```python
from build123d import *

# Parameters (mm, degrees)
SKETCH1_R           = 1.65
SKETCH1_R_2         = 9.5
BOSS_EXTRUDE1_DEPTH = 1


with BuildPart() as part:
    # Sketch1 → Boss-Extrude1 (new body)
    with BuildSketch(Plane.XY):
        with BuildLine():
            ThreePointArc((10.142857143, 9.649997356), (9, 15.588457268), (3.285714286, 13.608970631))
            ThreePointArc((3.285714286, 13.608970631), (-7, 12.124355653), (-13.428571429, 3.958973274))
            ThreePointArc((-13.428571429, 3.958973274), (-18, 0), (-13.428571429, -3.958973274))
            ThreePointArc((-13.428571429, -3.958973274), (-7, -12.124355653), (3.285714286, -13.608970631))
            ThreePointArc((3.285714286, -13.608970631), (9, -15.588457268), (10.142857143, -9.649997356))
            ThreePointArc((10.142857143, -9.649997356), (14, 0), (10.142857143, 9.649997356))
        make_face()
        with Locations((7, 12.124355653)):
            Circle(SKETCH1_R, mode=Mode.SUBTRACT)
        with Locations((7, -12.124355653)):
            Circle(SKETCH1_R, mode=Mode.SUBTRACT)
        with Locations((-14, 0)):
            Circle(SKETCH1_R, mode=Mode.SUBTRACT)
        Circle(SKETCH1_R_2, mode=Mode.SUBTRACT)
    extrude(amount=BOSS_EXTRUDE1_DEPTH)


solid = part.part
```
Model file for the job. Use its own axes, mm. Coordinates: 2 decimals unless noted, no trailing zeros. Order: outer loops, then holes, each group sorted by start corner. A loop starts at its lowest first (then second) coordinate and runs counter-clockwise, first axis right, second up. Notation, with made-up numbers: (74, -8) -> (117, -8) arc R24 ccw to (117, 20) -> close; hole circle Ø10 at (62.5, 43.25). An arc over 180 degrees is marked (long way). Answer as a JSON object with one key per item and string values. Group by question number.
1) Cut at C-C, the plane y = 0. Write the cut outline in (x, z).
2) Cut at D-D, the plane x = 7. Write the cut outline in (y, z), then the cut area to 3 significant figures.
3) Pull direction Y, two halves, no side cores. Call faces 1 (the face through (-12.476, -0.632, 0.493)), 2 (the face through (6.79, 13.76, 0.49)), 3 (the face through (-7.13, -12.05, 0.49)), 4 (the face through (0, 10, 1)): +Y half, -Y half, draft (parallel to the pull), parting line (faces both ways), or undercut.
4) Cut at A-A, the plane x = -14. Write the cut outline in (y, z), then the cut area to 3 significant figures.
5) Cut at B-B, the plane y = -9. Write the cut outline in (x, z), then the cut area to 3 significant figures.
6) Drill centre lines: L1, parallel to Y at x = 7, z = 0.65; L2, parallel to Y at x = 0, z = 0.45; L3, parallel to Y at x = -14, z = 0.7. Where is each one in solid material? Low to high.
Check values:
{
 "1": {"outline": "(-18, 0) -> (-15.65, 0) -> (-15.65, 1) -> (-18, 1) -> close; (-12.35, 0) -> (-9.5, 0) -> (-9.5, 1) -> (-12.35, 1) -> close; (9.5, 0) -> (14, 0) -> (14, 1) -> (9.5, 1) -> close"},
 "2": {"outline": "(-16.12, 0) -> (-13.77, 0) -> (-13.77, 1) -> (-16.12, 1) -> close; (-10.47, 0) -> (-6.42, 0) -> (-6.42, 1) -> (-10.47, 1) -> close; (6.42, 0) -> (10.47, 0) -> (10.47, 1) -> (6.42, 1) -> close; (13.77, 0) -> (16.12, 0) -> (16.12, 1) -> (13.77, 1) -> close", "area": "12.8 mm²"},
 "3": {"face 1": "undercut", "face 2": "undercut", "face 3": "-Y half", "face 4": "draft"},
 "4": {"outline": "(-4, 0) -> (-1.65, 0) -> (-1.65, 1) -> (-4, 1) -> close; (1.65, 0) -> (4, 0) -> (4, 1) -> (1.65, 1) -> close", "area": "4.70 mm²"},
 "5": {"outline": "(-10.72, 0) -> (-3.04, 0) -> (-3.04, 1) -> (-10.72, 1) -> close; (3.04, 0) -> (10.72, 0) -> (10.72, 1) -> (3.04, 1) -> close", "area": "15.4 mm²"},
 "6": {"L1": "y = -16.12 to -13.77, -10.47 to -6.42, 6.42 to 10.47, 13.77 to 16.12", "L2": "y = -14 to -9.5, 9.5 to 14", "L3": "y = -4 to -1.65, 1.65 to 4"}
}
